Check sheet for the modelled part. Datum: model origin and axes. Units: mm. Face numbers are marked on the shaded views. A direction names the side the tool comes from. Coordinates: 2 decimals unless noted, no trailing zeros. Loops run counter-clockwise (first coordinate to the right, second up) from the corner with the lowest first, then second, coordinate; pieces in that order, holes last. Notation, with made-up numbers: M 34,59 L 40,59 A25 ccw 40,97 Z; hole C 88.25,27.25 d6. An arc over 180 degrees is marked long. Answer in a Markdown table with one row per item. Add a question column.
```python
from build123d import *

# Parameters (mm, degrees)
EXTRUDE_1_DEPTH = 1.5
SKETCH_2_W      = 30
SKETCH_2_H      = 27.5
EXTRUDE_2_DEPTH = 6.5
SKETCH_3_W      = 13.2
SKETCH_3_H      = 21.5
EXTRUDE_3_DEPTH = 12
SKETCH_4_W      = 3.188486523
SKETCH_4_H      = 10
EXTRUDE_4_DEPTH = 3.5


with BuildPart() as part:
    # 草图1 → 凸台-拉伸1 (new body)
    with BuildSketch(Plane(origin=(0, 0, 0), x_dir=(1, 0, 0), z_dir=(0, 1, 0))):
        Polygon((-23.5, 10.75), (-12.5, 10.75), (-12.5, 13.75), (23.5, 13.75), (23.5, -13.75), (-12.5, -13.75), (-12.5, -10.75), (-23.5, -10.75), align=None)
    extrude(amount=EXTRUDE_1_DEPTH)

    # 草图2 → 凸台-拉伸2 (add)
    with BuildSketch(Plane(origin=(0, 1.5, 0), x_dir=(1, 0, 0), z_dir=(0, 1, 0))):
        with Locations((2.5, 0)):
            Rectangle(SKETCH_2_W, SKETCH_2_H)
    extrude(amount=EXTRUDE_2_DEPTH)

    # 草图3 → 凸台-拉伸3 (add)
    with BuildSketch(Plane(origin=(0, 1.5, 0), x_dir=(1, 0, 0), z_dir=(0, 1, 0))):
        with Locations((-19.1, 0)):
            Rectangle(SKETCH_3_W, SKETCH_3_H)
    extrude(amount=EXTRUDE_3_DEPTH)

    # 草图4 → 凸台-拉伸4 (add)
    with BuildSketch(Plane(origin=(0, 1.5, 0), x_dir=(1, 0, 0), z_dir=(0, 1, 0))):
        with Locations((21.905756739, 6.25)):
            Rectangle(SKETCH_4_W, SKETCH_4_H)
        with Locations((21.905756739, -6.25)):
            Rectangle(SKETCH_4_W, SKETCH_4_H)
    extrude(amount=EXTRUDE_4_DEPTH)


solid = part.part
```
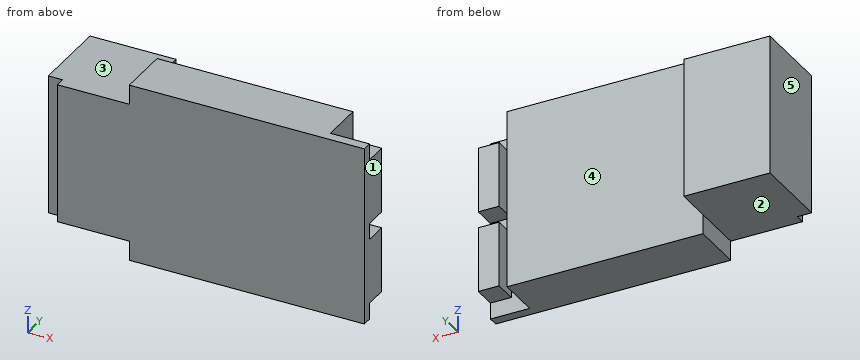
Q1. Access from +Z, -Z, +X, -X, +Y, -Y to the whole of each face (thin tool, end or side, straight path). Record for the marked faces 1, 2, 3, 4 and 5.
Q2. Go/stop test with flat-tipped pins: pin 1 (5 mm diameter, centred on x = -19, y = 12, fed in from -Z); pin 2 (3.5 mm diameter, centred on x = 21.5, y = 4, fed in from +Z); pin 3 (1 mm diameter, centred on x = -17.5, z = 7, fed in from -Y); pin 4 (4 mm diameter, centred on y = 7.5, z = 5, fed in from +X). Record where each tip stops, or that it passes through.
Q3. Cross-section at C-C (y = 5.5). Record the cut outline in (x, z).
Q4. Cross-section at D-D (x = -14). Record the cut outline in (y, z), plus the area to 3 significant figures.
Q5. Thickness scan on L1, parallel to X at y = 2, z = -2; L2, parallel to Z at x = -17.5, y = 9; L3, parallel to X at y = 9.5, z = -4.5. Record the ranges inside material, lowest first.
Q6. Cross-section at B-B (z = -5.75). Record the cut outline in (x, y), plus the area to 3 significant figures.
Q7. Cross-section at A-A (y = 2). Record the cut outline in (x, z).
Answer key:
| question | item | result |
|---|---|---|
| 1 | face 1 | +Z, -Z, +X, +Y, -Y |
| 1 | face 2 | -Z, -X, +Y, -Y |
| 1 | face 3 | +Z, -X, +Y, -Y |
| 1 | face 4 | +Z, -Z, +X, +Y |
| 1 | face 5 | +Z, -Z, -X, +Y, -Y |
| 2 | pin 1 | z = -10.75 |
| 2 | pin 2 | z = 11.25 |
| 2 | pin 3 | y = 0 |
| 2 | pin 4 | x = 17.5 |
| 3 | outline | M -25.7,-10.75 L -12.5,-10.75 L -12.5,-13.75 L 17.5,-13.75 L 17.5,13.75 L -12.5,13.75 L -12.5,10.75 L -25.7,10.75 Z |
| 4 | outline | M 0,-10.75 L 13.5,-10.75 L 13.5,10.75 L 0,10.75 Z |
| 4 | area | 290 mm^2 |
| 5 | L1 | -25.7 to 17.5, 20.31 to 23.5 |
| 5 | L2 | -10.75 to 10.75 |
| 5 | L3 | -25.7 to -12.5 |
| 6 | outline | M -25.7,1.5 L -23.5,1.5 L -23.5,0 L 23.5,0 L 23.5,5 L 20.31,5 L 20.31,1.5 L 17.5,1.5 L 17.5,8 L -12.5,8 L -12.5,13.5 L -25.7,13.5 Z |
| 6 | area | 435 mm^2 |
| 7 | outline | M -25.7,-10.75 L -12.5,-10.75 L -12.5,-13.75 L 17.5,-13.75 L 17.5,13.75 L -12.5,13.75 L -12.5,10.75 L -25.7,10.75 Z; M 20.31,-11.25 L 23.5,-11.25 L 23.5,-1.25 L 20.31,-1.25 Z; M 20.31,1.25 L 23.5,1.25 L 23.5,11.25 L 20.31,11.25 Z |
